Part print with two shaded views. Sizes in mm from the minimum x, y, z corner. A direction names the side the tool comes from. Coordinates: 2 decimals unless noted, no trailing zeros. Write each loop counter-clockwise with the first axis right and the second up, starting at its lowest first coordinate (ties: lowest second). Pieces come first, ordered by that corner, then holes. Notation, with made-up numbers: (40.5, 0.5) - (95.5, 0.5) arc R24 cw to (95.5, 14.5) - close; hole circle Ø11 at (36.5, 74.25). An arc over 180 degrees is marked (long way). Answer in a Markdown table with one row per item. Add a question column.
Q1. Band-saw the part on A-A (x = 5.1). List the corners of the cut face in (y, z).
Q2. 3-axis set-ups, long thin cutter, end or side, ignore diameter. For the marked faces 5 and 6: which of +Z, -Z, +X, -X, +Y, -Y reach the whole face in a straight line?
Q3. Band-saw the part on D-D (x = 14.6). List the corners of the cut face in (y, z).
Q4. Drill centre lines: line 1 along Y through (x, z) = (14.6, 2.3); line 2 along Y through (x, z) = (5.1, 1.05); line 3 along X through (y, z) = (3.75, 4.05) (1 decimal). Where is each one in solid material? Low to high. Write a range as from..to.
Q5. Two-plate mould, pull along X, no slides. Class the marked faces 1, 2, 3 and 4: +X half, -X half, draft (parallel to the pull), parting line (faces both ways), or undercut.
Q6. Band-saw the part on B-B (y = 2.9). List the corners of the cut face in (x, z).
Q7. Band-saw the part on C-C (z = 3.9). List the corners of the cut face in (x, y), and give its area (3 significant figures).
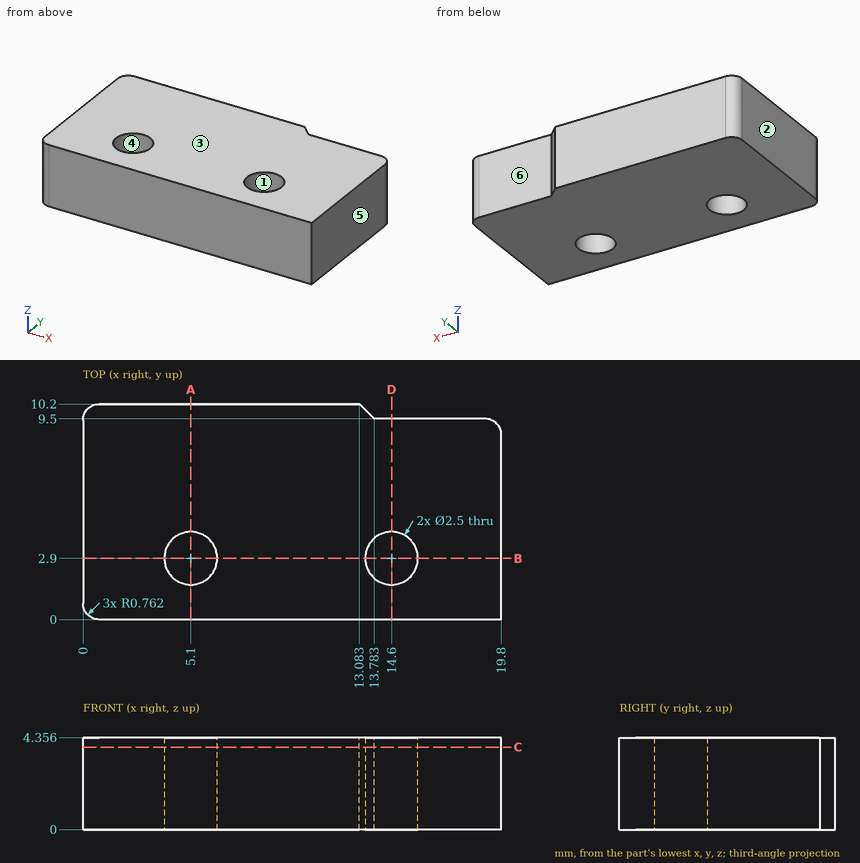
Checked values:
| question | item | result |
|---|---|---|
| 1 | outline | (0, 0) - (1.65, 0) - (1.65, 4.36) - (0, 4.36) - close; (4.15, 0) - (10.2, 0) - (10.2, 4.36) - (4.15, 4.36) - close |
| 2 | face 5 | +Z, -Z, +X, +Y, -Y |
| 2 | face 6 | +Z, -Z, +X, +Y |
| 3 | outline | (0, 0) - (1.65, 0) - (1.65, 4.36) - (0, 4.36) - close; (4.15, 0) - (9.5, 0) - (9.5, 4.36) - (4.15, 4.36) - close |
| 4 | line 1 | y = 0..1.65, 4.15..9.5 |
| 4 | line 2 | y = 0..1.65, 4.15..10.2 |
| 4 | line 3 | x = 0..4.2, 6..13.7, 15.5..19.8 |
| 5 | face 1 | undercut |
| 5 | face 2 | -X half |
| 5 | face 3 | draft |
| 5 | face 4 | undercut |
| 6 | outline | (0, 0) - (3.85, 0) - (3.85, 4.36) - (0, 4.36) - close; (6.35, 0) - (13.35, 0) - (13.35, 4.36) - (6.35, 4.36) - close; (15.85, 0) - (19.8, 0) - (19.8, 4.36) - (15.85, 4.36) - close |
| 7 | outline | (0, 0.76) arc R0.76 ccw to (0.76, 0) - (19.8, 0) - (19.8, 8.74) arc R0.76 ccw to (19.04, 9.5) - (13.78, 9.5) - (13.08, 10.2) - (0.76, 10.2) arc R0.76 ccw to (0, 9.44) - close; hole circle Ø2.5 at (5.1, 2.9); hole circle Ø2.5 at (14.6, 2.9) |
| 7 | area | 187 mm² |
